from build123d import *

# Parameters (mm, degrees)
ESTRUSIONE_ESTRUSIONE2_DEPTH = 20
FORO_PER_VITE_M4_2_D         = 4.5
FORO_PER_VITE_M4_2_DEPTH     = 15
FORO_PER_VITE_M4_2_TIP       = 1.351936393
SCHIZZO6_R                   = 7.5
TAGLIO_ESTRUSIONE1_DEPTH     = 3
FORO_PER_VITE_M4_1_D         = 4
FORO_PER_VITE_M4_1_DEPTH     = 9
FORO_PER_VITE_M4_1_TIP       = 1.201721238


with BuildPart() as part:
    # Schizzo2 → Estrusione-Estrusione2 (new body)
    with BuildSketch(Plane(origin=(0, 0, 0), x_dir=(1, 0, 0), z_dir=(0, 1, 0))):
        Polygon((5, 30), (5, 10.303300859), (10.303300859, 5), (30, 5), (30, 0), (0, 0), (0, 30), align=None)
    extrude(amount=ESTRUSIONE_ESTRUSIONE2_DEPTH)

    # Foro per Vite M4-2
    with Locations(Plane(origin=(5, 0, 0), x_dir=(0, 0, -1), z_dir=(1, 0, 0))):
        with Locations((17.5, 10)):
            Hole(FORO_PER_VITE_M4_2_D / 2, depth=FORO_PER_VITE_M4_2_DEPTH)
            with Locations((0, 0, -(FORO_PER_VITE_M4_2_DEPTH + FORO_PER_VITE_M4_2_TIP / 2))):  # 118° drill point
                Cone(0, FORO_PER_VITE_M4_2_D / 2, FORO_PER_VITE_M4_2_TIP, mode=Mode.SUBTRACT)

    # Schizzo6 → Taglio-Estrusione1 (cut)
    with BuildSketch(Plane.XY):
        with Locations((20, 10)):
            Circle(SCHIZZO6_R)
    extrude(amount=-TAGLIO_ESTRUSIONE1_DEPTH, mode=Mode.SUBTRACT)

    # Foro per Vite M4-1
    with Locations(Plane(origin=(20, 10, 0), x_dir=(1, 0, 0), z_dir=(0, 0, 1))):
        with Locations((0, 0)):
            Hole(FORO_PER_VITE_M4_1_D / 2, depth=FORO_PER_VITE_M4_1_DEPTH)
            with Locations((0, 0, -(FORO_PER_VITE_M4_1_DEPTH + FORO_PER_VITE_M4_1_TIP / 2))):  # 118° drill point
                Cone(0, FORO_PER_VITE_M4_1_D / 2, FORO_PER_VITE_M4_1_TIP, mode=Mode.SUBTRACT)


solid = part.part
For this review, take the finished solid that the model builds, in its own axes (mm). A direction names the side the tool comes from. Give positions to 0.01 mm unless a question says otherwise; leave off trailing zeros. Loops run counter-clockwise (first coordinate to the right, second up) from the corner with the lowest first, then second, coordinate; pieces in that order, holes last. Notation, with made-up numbers: M 10.5,2.5 L 31.5,2.5 A15 cw 31.5,6.5 Z; hole C 2.5,61 d9. An arc over 180 degrees is marked long. Answer as a JSON object with one key per item and string values. Group by question number.
Q1. Tool access review of faces 5 (the flat face through (2, 10, -30)), 6 (the cylindrical face through (14.048, 5.436, -1.479)): name each direction out of +Z, -Z, +X, -X, +Y, -Y from which nothing blocks a thin tool from reaching the whole face with its end or side.
Q2. Mouldability with a two-part tool opening along X and no side actions: class faces 1 (the flat face through (22, 8, -3)), 2 (the flat face through (5, 10, -20)), 3 (the flat face through (17.8, 9.9, -5)), 4 (the flat face through (0, 10, -15)) as +X half, -X half, draft (parallel to the pull), parting line (faces both ways), or undercut.
Q3. Insertion check: P1, Ø12, axis at x = 20, y = 10, coming from the +Z side; P2, Ø6, axis at x = 14.5, y = 11, coming from the -Z side; P3, Ø2, axis at y = 15.5, z = -13, coming from the +X side. Each pin has a flat end and moves straight along its axis. Give the tip position at first contact, or say it passes through.
Q4. Add section D-D on y = 6.25. Give the boundary of the cut face in (x, z), and give its area (3 significant figures).
Q5. Add section A-A on z = -17.5. Give the boundary of the cut face in (x, y), and give its area (3 significant figures).
Q6. Add section B-B on x = 20. Give the boundary of the cut face in (y, z), and give its area (3 significant figures).
Q7. For probe 1 along Y at (x, z) = (20, -0.8); probe 2 along Y at (x, z) = (2.05, -17.5); probe 3 along X at (y, z) = (3.25, -13), list the stretches that pass through material, from the lowest coordinate up. Write a range as [from, to].
Q8. Add section C-C on y = 8.75. Give the boundary of the cut face in (x, z), and give its area (3 significant figures).
Checked values:
{
 "1": {"face 5": "-Z, +X, -X, +Y, -Y", "face 6": "+Z"},
 "2": {"face 1": "undercut", "face 2": "+X half", "face 3": "draft", "face 4": "-X half"},
 "3": {"P1": "z = -3", "P2": "z = -5", "P3": "x = 5"},
 "4": {"outline": "M 0,-30 L 5,-30 L 5,-10.3 L 10.3,-5 L 30,-5 L 30,0 L 26.5,0 L 26.5,-3 L 13.5,-3 L 13.5,0 L 0,0 Z", "area": "250 mm²"},
 "5": {"outline": "M 0,0 L 5,0 L 5,7.75 L 0,7.75 Z; M 0,12.25 L 5,12.25 L 5,20 L 0,20 Z", "area": "77.5 mm²"},
 "6": {"outline": "M 0,-5 L 8,-5 L 8,-3 L 2.5,-3 L 2.5,0 L 0,0 Z; M 12,-5 L 20,-5 L 20,0 L 17.5,0 L 17.5,-3 L 12,-3 Z", "area": "47.0 mm²"},
 "7": {"probe 1": "[0, 2.5], [17.5, 20]", "probe 2": "[0, 7.75], [12.25, 20]", "probe 3": "[0, 5]"},
 "8": {"outline": "M 0,-30 L 5,-30 L 5,-19.37 L 0,-19.37 Z; M 0,-15.63 L 5,-15.63 L 5,-10.3 L 10.3,-5 L 18.44,-5 L 18.44,-3 L 12.6,-3 L 12.6,0 L 0,0 Z; M 21.56,-5 L 30,-5 L 30,0 L 27.4,0 L 27.4,-3 L 21.56,-3 Z", "area": "220 mm²"}
}
